Autodesk Inventor part; units mm, degrees
ref_plane "YZ Plane" through (0, 0, 0) normal (1, 0, 0) x (0, 1, 0)
ref_plane "XZ Plane" through (0, 0, 0) normal (0, 1, 0) x (-1, 0, 0)
ref_plane "XY Plane" through (0, 0, 0) normal (0, 0, 1) x (1, 0, 0)
sketch "Sketch1" plane through (0, 0, 0) normal (0, 0, 1) x (1, 0, 0)
  circle A0 centre (0, 0) radius 15.875
  line L0 (-38.1, 0) -> (-38.1, -6.35)
  line L1 (-38.1, 0) -> (-38.1, 6.35)
  line L2 (38.1, 0) -> (38.1, 6.35)
  line L3 (38.1, 0) -> (38.1, -6.35)
  line L4 (-38.1, 6.35) -> (-63.1817, 6.35)
  line L5 (-38.1, -6.35) -> (-63.1817, -6.35)
  line L6 (38.1, 6.35) -> (63.1817, 6.35)
  line L7 (38.1, -6.35) -> (63.1817, -6.35)
  line L8 (0, 38.1) -> (6.35, 38.1)
  line L9 (6.35, 38.1) -> (6.35, 63.1817)
  line L10 (0, 38.1) -> (-6.35, 38.1)
  line L11 (-6.35, 38.1) -> (-6.35, 63.1817)
  line L12 (0, 0) -> (0, -38.1)
  line L13 (0, -38.1) -> (6.35, -38.1)
  line L14 (0, -38.1) -> (-6.35, -38.1)
  line L15 (-6.35, -38.1) -> (-6.35, -63.1817)
  line L16 (6.35, -38.1) -> (6.35, -63.1817)
  line L17 (-31.75, 38.1) -> (-31.75, 54.9926)
  line L18 (31.75, 38.1) -> (31.75, 54.9926)
  line L19 (38.1, 31.75) -> (54.9926, 31.75)
  line L20 (38.1, -31.75) -> (54.9926, -31.75)
  line L21 (31.75, -38.1) -> (31.75, -54.9926)
  line L22 (-31.75, -38.1) -> (-31.75, -54.9926)
  line L23 (-38.1, 31.75) -> (-54.9926, 31.75)
  line L24 (-38.1, -31.75) -> (-54.9926, -31.75)
  line L25 (-38.1, -31.75) -> (-31.75, -31.75)
  line L26 (-31.75, -31.75) -> (-31.75, -38.1)
  line L27 (31.75, -38.1) -> (31.75, -31.75)
  line L28 (31.75, -31.75) -> (38.1, -31.75)
  arc A1 (-6.35, 63.1817) -> (-31.75, 54.9926) centre (0, 0) ccw
  arc A2 (31.75, 54.9926) -> (6.35, 63.1817) centre (0, 0) ccw
  arc A3 (63.1817, 6.35) -> (54.9926, 31.75) centre (0, 0) ccw
  arc A4 (6.35, -63.1817) -> (31.75, -54.9926) centre (0, 0) ccw
  arc A5 (54.9926, -31.75) -> (63.1817, -6.35) centre (0, 0) ccw
  arc A6 (-31.75, -54.9926) -> (-6.35, -63.1817) centre (0, 0) ccw
  arc A7 (-54.9926, 31.75) -> (-63.1817, 6.35) centre (0, 0) ccw
  arc A8 (-63.1817, -6.35) -> (-54.9926, -31.75) centre (0, 0) ccw
  line L29 (31.75, 38.1) -> (31.75, 31.75)
  line L30 (31.75, 31.75) -> (38.1, 31.75)
  line L31 (-38.1, 31.75) -> (-31.75, 31.75)
  line L32 (-31.75, 31.75) -> (-31.75, 38.1)
  dimension "d6" = 31.75
  dimension "d7" = 38.1
  dimension "d8" = 38.1
  dimension "d9" = 6.35
  dimension "d10" = 6.35
  dimension "d11" = 6.35
  dimension "d12" = 6.35
  dimension "d14" = 6.35
  dimension "d15" = 6.35
  dimension "d16" = 38.1
  dimension "d17" = 6.35
  dimension "d18" = 25.4
  dimension "d19" = 25.4
  dimension "d20" = 25.4
  dimension "d22" = 25.4
  dimension "d23" = 25.4
  dimension "d24" = 25.4
  dimension "d25" = 25.4
extrude "Extrusion1" add sketch "Sketch1" along normal blind 25.4
sketch "Sketch2" plane through (0, 0, 25.4) normal (0, 0, 1) x (1, 0, 0)
  circle A0 centre (0, 0) radius 15.875
  circle A1 centre (0, 0) radius 28.575
  dimension "d28" = 31.75
  dimension "d29" = 57.15
extrude "Extrusion2" add sketch "Sketch2" along normal blind 19.05
properties part number "Assignment 3.5 - Indexing Guide"
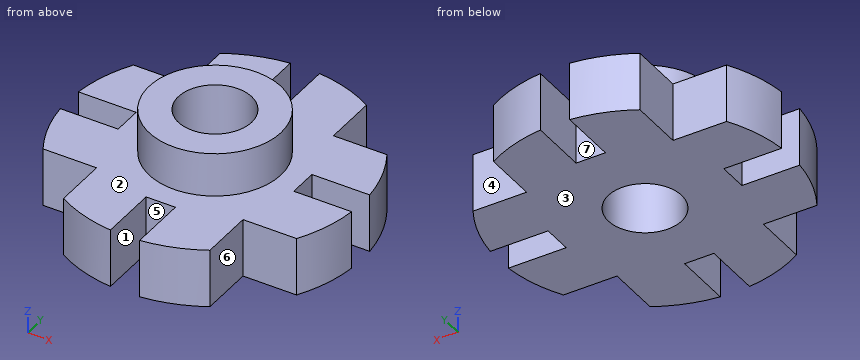
Verification items for the finished model (mm, model axes). Face numbers are marked on the shaded views. A direction names the side the tool comes from. Give positions to 0.01 mm unless a question says otherwise; leave off trailing zeros. Loops run counter-clockwise (first coordinate to the right, second up) from the corner with the lowest first, then second, coordinate; pieces in that order, holes last.
1) Depth check by flat-ended pin: pin 1 Ø4 at (y, z) = (-11.5, 17) entering from +X; pin 2 Ø14 at (y, z) = (2, 9) entering from +X; pin 3 Ø7 at (x, z) = (46.5, 17.5) entering from +Y; pin 4 Ø12 at (x, y) = (-43.5, -40.5) entering from -Z. Enter the tip coordinate at first touch or a pass-through.
2) Thickness scan on line 1 along Y through (x, z) = (0, 18) (3 decimals); line 2 along Y through (x, z) = (0, 31) (3 decimals); line 3 along X through (y, z) = (48, 19). Record the ranges inside material, lowest first.
3) Sectioned sample at A-A, the plane y = 0. Enter the section's corners in (x, z) (3 decimals).
4) Draft check along Z on the marked faces 1, 2 and 3. Enter one of: pulls with the +Z half, pulls with the -Z half, needs draft (parallel to the pull), parting line crosses it, or undercut.
5) Set-up check for the marked faces 4, 5, 6 and 7: record each of +Z, -Z, +X, -X, +Y, -Y from which the full face is reachable in a straight line by a thin tool's end or side.
6) Sectioned sample at B-B, the plane x = -40. Enter the section's corners in (y, z).
Answers:
1. pin 1: stops at x = 62.79
1. pin 2: stops at x = 63.18
1. pin 3: stops at y = 31.75
1. pin 4: passes through
2. line 1: y = -38.1 to -15.875, 15.875 to 38.1
2. line 2: y = -28.575 to -15.875, 15.875 to 28.575
2. line 3: x = -31.75 to -6.35, 6.35 to 31.75
3. outline: (-38.1, 0) - (-15.875, 0) - (-15.875, 44.45) - (-28.575, 44.45) - (-28.575, 25.4) - (-38.1, 25.4) - close; (15.875, 0) - (38.1, 0) - (38.1, 25.4) - (28.575, 25.4) - (28.575, 44.45) - (15.875, 44.45) - close
4. face 1: needs draft
4. face 2: pulls with the +Z half
4. face 3: pulls with the -Z half
5. face 4: +Z, -Z, +X, +Y
5. face 5: +Z, -Z, -Y
5. face 6: +Z, -Z, +X, -Y
5. face 7: +Z, -Z, +Y
6. outline: (-31.75, 0) - (-6.35, 0) - (-6.35, 25.4) - (-31.75, 25.4) - close; (6.35, 0) - (31.75, 0) - (31.75, 25.4) - (6.35, 25.4) - close
